Design review of the part built by this model. Coordinates are the model's own, in mm. Face numbers are marked on the shaded views. A direction names the side the tool comes from. Give positions to 0.01 mm unless a question says otherwise; leave off trailing zeros. Order: outer loops, then holes, each group sorted by start corner. A loop starts at its lowest first (then second) coordinate and runs counter-clockwise, first axis right, second up. Notation, with made-up numbers: (80, -13) -> (112, -13) arc R24 cw to (112, 17) -> close; hole circle Ø5 at (41.5, -19). An arc over 180 degrees is marked (long way). One line per item, written item: value. Start each with the question number.
1) Consider section B-B (x = -32.75). State the section outline as (y, z) points, plus the area to 3 significant figures.
2) Consider section A-A (z = -19). State the section outline as (x, y) points.
3) Tool access review of the marked faces 1, 2 and 3: name each direction out of +Z, -Z, +X, -X, +Y, -Y from which nothing blocks a thin tool from reaching the whole face with its end or side.
4) Wall thickness on line 1 along Y through (x, z) = (-33.5, -9); line 2 along X through (y, z) = (23.5, -14.5); line 3 along Y through (x, z) = (-24.25, -4): over which ranges is each line inside the solid? List them lowest first. Write a range as from..to.
5) Consider section C-C (y = 8). State the section outline as (x, z) points.
6) For pin 1 (3 mm diameter, centred on y = 27, z = -17, fed in from +X); pin 2 (7 mm diameter, centred on x = -16.5, z = 3.5, fed in from +Y); pin 3 (1.5 mm diameter, centred on y = 28.5, z = -14.5, fed in from -X); pin 4 (5 mm diameter, centred on x = -19, y = -1.5, fed in from -Z), all flat-tipped, find the tip position at first contact; note any pin that passes through.
from build123d import *

# Parameters (mm, degrees)
F0_W     = 7.9843644053
F0_H     = 67.8671114147
F1_DEPTH = 6.35
F2_DEPTH = 7.62
F3_DEPTH = 25.4


with BuildPart() as f1:
    # F0 (on Top) → F1 (new body)
    with BuildSketch(Plane.XY):
        with Locations((-27.2799162194, 10.146798566)):
            Rectangle(F0_W, F0_H)
        with BuildLine():
            ThreePointArc((-23.2877340168, 44.0803542733), (-27.2799162194, 48.072536476), (-31.2720984221, 44.0803542733))
            Line((-31.2720984221, 44.0803542733), (-23.2877340168, 44.0803542733))
        make_face()
        Polygon((-34.5989204943, -23.7867571414), (-34.5989204943, -75.3524526954), (-18.9628694206, -75.3524526954), (-18.9628694206, -23.7867571414), (-23.2877340168, -23.7867571414), (-31.2720984221, -23.7867571414), align=None)
    extrude(amount=F1_DEPTH)

    # F2 (add): a face of the model
    f2_faces = [f1.faces().sort_by_distance(p)[0] for p in [
        (-18.9628694206, -49.5696049184, 3.175),
    ]]
    extrude(f2_faces, amount=F2_DEPTH)

    # F3 (add): a face of the model
    f3_faces = [f1.faces().sort_by_distance(p)[0] for p in [
        (-24.3540524425, -29.8961498867, 0),
    ]]
    extrude(f3_faces, amount=F3_DEPTH)


solid = f1.part
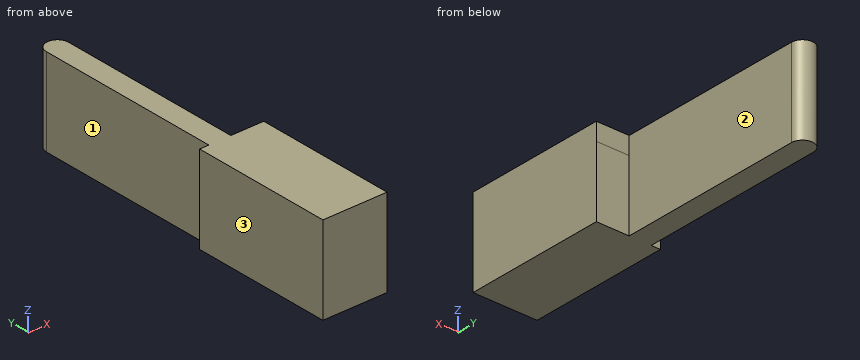
Checked values:
1. outline: (-75.35, -25.4) -> (-23.79, -25.4) -> (-23.79, 6.35) -> (-75.35, 6.35) -> close
1. area: 1,640 mm^2
2. outline: (-34.6, -75.35) -> (-11.34, -75.35) -> (-11.34, -23.79) -> (-23.29, -23.79) -> (-23.29, 44.08) arc R3.99 ccw to (-31.27, 44.08) -> (-31.27, -23.79) -> (-34.6, -23.79) -> close
3. face 1: +Z, -Z, -X, +Y
3. face 2: +Z, -Z, +X, +Y
3. face 3: +Z, -Z, -X, +Y, -Y
4. line 1: y = -75.35..-23.79
4. line 2: x = -31.27..-23.29
4. line 3: y = -75.35..46.68
5. outline: (-31.27, -25.4) -> (-23.29, -25.4) -> (-23.29, 6.35) -> (-31.27, 6.35) -> close
6. pin 1: stops at x = -23.29
6. pin 2: stops at y = -23.79
6. pin 3: stops at x = -31.27
6. pin 4: passes through
